Work out the finished part from the listing and answer in its coordinate system (mm). Round coordinates to 2 decimals unless told otherwise and drop trailing zeros. Write each loop counter-clockwise with the first axis right and the second up, starting at its lowest first coordinate (ties: lowest second). Pieces come first, ordered by that corner, then holes.
1. Straight lines are drawn through the part: probe 1 along Z at (x, y) = (10, -6.5); probe 2 along X at (y, z) = (-7.5, -0.5); probe 3 along X at (y, z) = (-3.75, -1). For each, find the intervals that lie inside material, in ascending order.
2. Find section B-B (x = -10). Write down the section's boundary in (y, z).
3. Find section A-A (z = 0). Write down the section's boundary in (x, y) (1 decimal).
4. Find section C-C (y = -8.75). Write down the section's boundary in (x, z).
5. A flat-ended cylindrical pin translates along its axis: pin 1 Ø1 at (x, z) = (-10.5, -1) entering from -Y. Find the tip coordinate at first contact, or state that the pin passes through.
6. Find section D-D (x = 10.75). Write down the section's boundary in (y, z), and give its area (3 significant figures).
```python
from build123d import *

# Parameters (mm, degrees)
SKETCH1_W            = 30
SKETCH1_H            = 8
BOSS_EXTRUDE1_DEPTH  = 10
M3_CLEARANCE_HOLE1_D = 3.4
CUT_EXTRUDE1_DEPTH   = 20.723082923


with BuildPart() as part:
    # Sketch1 → Boss-Extrude1 (new body)
    with BuildSketch(Plane(origin=(0, 0, 0), x_dir=(1, 0, 0), z_dir=(0, 1, 0))):
        Rectangle(SKETCH1_W, SKETCH1_H)
    extrude(amount=-BOSS_EXTRUDE1_DEPTH)

    # M3 Clearance Hole1 (through all)
    with Locations(Plane(origin=(0, 0, 0), x_dir=(-1, 0, 0), z_dir=(0, 1, 0))):
        with Locations((10, 0), (-10, 0)):
            Hole(M3_CLEARANCE_HOLE1_D / 2)

    # Sketch2 → Cut-Extrude1 (cut, through all)
    with BuildSketch(Plane.XY.offset(4)):
        with BuildLine():
            Line((-4.736180555, 0), (4.736180555, 0))
            ThreePointArc((4.736180555, 0), (0, -4.2625), (-4.736180555, 0))
        make_face()
    extrude(amount=-CUT_EXTRUDE1_DEPTH, mode=Mode.SUBTRACT)


solid = part.part
```
Worked answers:
1. probe 1: z = -4 to -1.7, 1.7 to 4
1. probe 2: x = -15 to -11.62, -8.38 to 8.38, 11.62 to 15
1. probe 3: x = -15 to -11.37, -8.63 to -2.15, 2.15 to 8.63, 11.37 to 15
2. outline: (-10, -4) - (0, -4) - (0, -1.7) - (-10, -1.7) - close; (-10, 1.7) - (0, 1.7) - (0, 4) - (-10, 4) - close
3. outline: (-15, -10) - (-11.7, -10) - (-11.7, 0) - (-15, 0) - close; (-8.3, -10) - (8.3, -10) - (8.3, 0) - (4.7, 0) arc R4.8 cw to (-4.7, 0) - (-8.3, 0) - close; (11.7, -10) - (15, -10) - (15, 0) - (11.7, 0) - close
4. outline: (-15, -4) - (15, -4) - (15, 4) - (-15, 4) - close; hole circle Ø3.4 at (-10, 0); hole circle Ø3.4 at (10, 0)
5. pin 1: passes through
6. outline: (-10, -4) - (0, -4) - (0, -1.53) - (-10, -1.53) - close; (-10, 1.53) - (0, 1.53) - (0, 4) - (-10, 4) - close
6. area: 49.5 mm2
